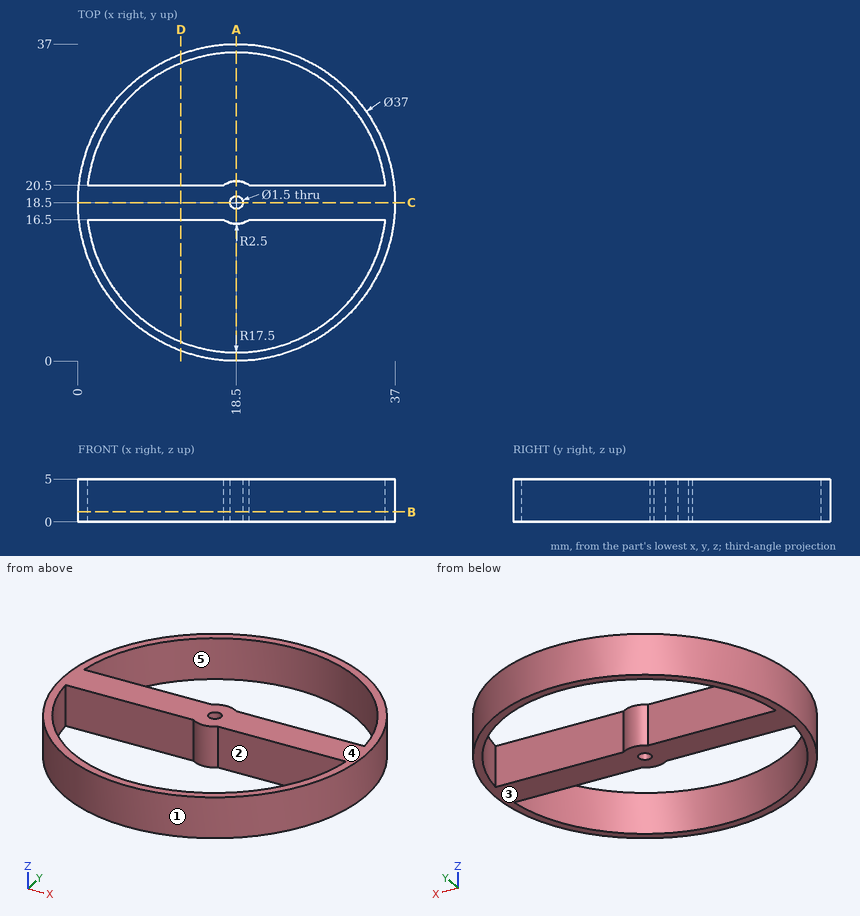
For this review, use the dimensioned drawing (mm, ordinates from the lowest corner) and the shaded views. A direction names the side the tool comes from. Coordinates: 2 decimals unless noted, no trailing zeros. Loops run counter-clockwise (first coordinate to the right, second up) from the corner with the lowest first, then second, coordinate; pieces in that order, holes last.
1. For line 1 (Y direction, x = 14.5, z = 0.6); line 2 (Y direction, x = 18, z = 2.9); line 3 (Y direction, x = 25.5, z = 3.45), list the stretches that pass through material, from the lowest coordinate up.
2. Add section A-A, the plane x = 18.5. Give the boundary of the cut face in (y, z).
3. For the marked faces 4 and 5, list the 3-axis set-ups (+Z, -Z, +X, -X, +Y, -Y) from which the entire face can be reached by the end or side of a thin tool; tool diameter is ignored.
4. Add section C-C, the plane y = 18.5. Give the boundary of the cut face in (x, z).
5. Add section D-D, the plane x = 12. Give the boundary of the cut face in (y, z).
6. Add section B-B, the plane z = 1.15. Give the boundary of the cut face in (x, y).
7. Mouldability with a two-part tool opening along X and no side actions: class the marked faces 1, 2 and 3 as +X half, -X half, draft (parallel to the pull), parting line (faces both ways), or undercut.
8. Insertion check: P1, Ø1.4, axis at x = 18.5, y = 18.5, coming from the -Z side (3 decimals); P2, Ø1.5, axis at x = 7.5, z = 2, coming from the +Y side; P3, Ø1.5, axis at y = 30, z = 2.5, coming from the -X side; P4, Ø1.5, axis at x = 25, z = 2, coming from the +Y side. Each pin has a flat end and moves straight along its axis. Give the tip position at first contact, or say it passes through.
Result:
1. line 1: y = 0.44 to 1.46, 16.5 to 20.5, 35.54 to 36.56
1. line 2: y = 0.01 to 1.01, 16.05 to 17.94, 19.06 to 20.95, 35.99 to 36.99
1. line 3: y = 1.38 to 2.46, 16.5 to 20.5, 34.54 to 35.62
2. outline: (0, 0) - (1, 0) - (1, 5) - (0, 5) - close; (16, 0) - (17.75, 0) - (17.75, 5) - (16, 5) - close; (19.25, 0) - (21, 0) - (21, 5) - (19.25, 5) - close; (36, 0) - (37, 0) - (37, 5) - (36, 5) - close
3. face 4: +Z, +X, -X, +Y, -Y
3. face 5: +Z, -Z
4. outline: (0, 0) - (17.75, 0) - (17.75, 5) - (0, 5) - close; (19.25, 0) - (37, 0) - (37, 5) - (19.25, 5) - close
5. outline: (1.18, 0) - (2.25, 0) - (2.25, 5) - (1.18, 5) - close; (16.5, 0) - (20.5, 0) - (20.5, 5) - (16.5, 5) - close; (34.75, 0) - (35.82, 0) - (35.82, 5) - (34.75, 5) - close
6. outline: circle Ø37 at (18.5, 18.5); hole (1.11, 16.5) arc R17.5 ccw to (35.89, 16.5) - (20, 16.5) arc R2.5 cw to (17, 16.5) - close; hole (1.11, 20.5) - (17, 20.5) arc R2.5 cw to (20, 20.5) - (35.89, 20.5) arc R17.5 ccw to start; hole circle Ø1.5 at (18.5, 18.5)
7. face 1: parting line
7. face 2: undercut
7. face 3: draft
8. P1: passes through
8. P2: stops at y = 33.9
8. P3: stops at x = 3.44
8. P4: stops at y = 36.08
